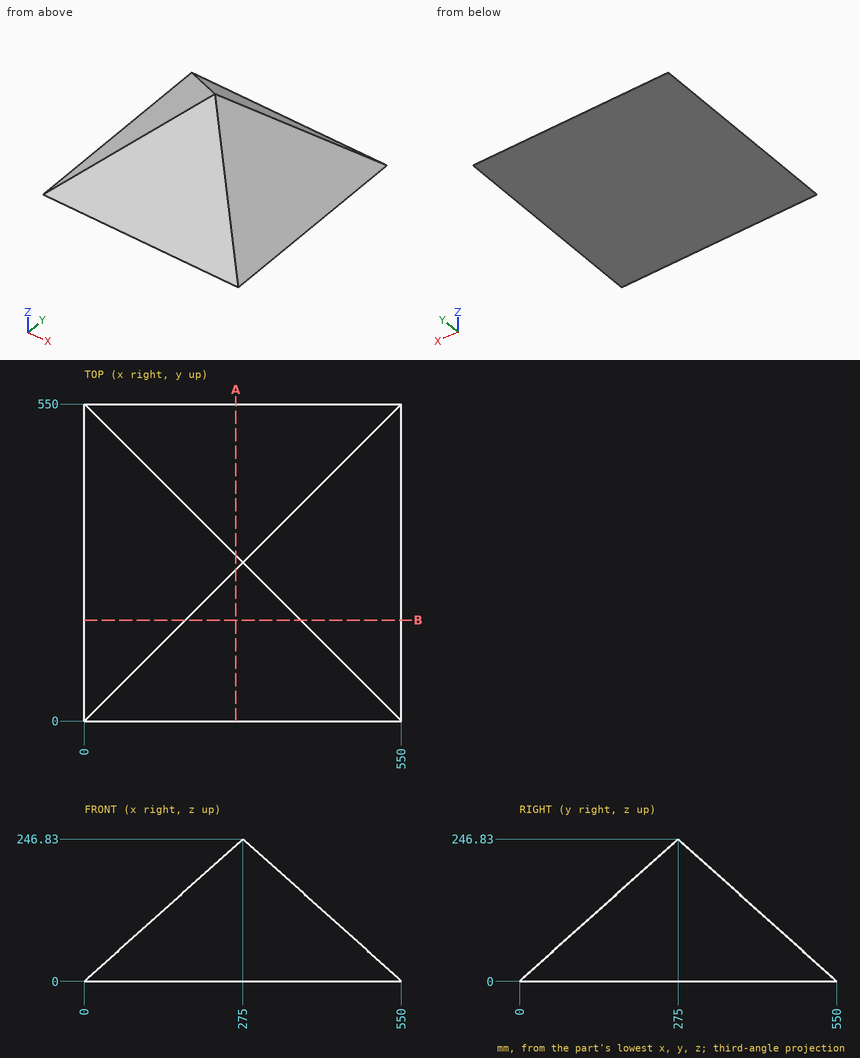
Could you check a few things on this drawing? It's one solid part, dimensions in mm from its lowest x, y, z. Give positions to 0.01 mm unless a question says otherwise; leave off trailing zeros. Write each loop counter-clockwise with the first axis right and the second up, starting at its lowest first coordinate (ties: lowest second). Pieces come first, ordered by that corner, then holes. Notation, with made-up numbers: (69, 57.5) -> (107, 57.5) arc R22 ccw to (107, 64.5) -> close; hole circle Ø8 at (-31.75, 85). An arc over 180 degrees is marked (long way). Write item = value, one per line.
(1) Suppose I cut it at A-A on x = 262.5. Write out the boundary of the cut face in (y, z), then the cut area to 3 significant figures.
Worked out:
outline = (0, 0) -> (550, 0) -> (287.5, 235.61) -> (262.5, 235.61) -> close
area = 67,700 mm^2
(2) I'm going to push flat-ended pins straight in: P1, Ø3, axis at x = 270, y = 366, coming from the +Z side; P2, Ø2, axis at y = 277.5, z = 218, coming from the -X side; P3, Ø6, axis at y = 286, z = 154, coming from the +X side. Where does each tip first touch, or does it pass through?
Worked out:
P1 = 166.5
P2 = 241.77
P3 = 381.77
(3) Suppose I cut it at B-B on y = 175. Write out the boundary of the cut face in (x, z).
Worked out:
outline = (0, 0) -> (550, 0) -> (375, 157.07) -> (175, 157.07) -> close
(4) I need wall thicknesses on probe 1 along Y at (x, z) = (177.5, 127); probe 2 along Z at (x, y) = (503.5, 255.5); probe 3 along Y at (x, z) = (290.5, 194). Which ranges of each line are inside material? Lowest first, please. Write a range as from..to.
Worked out:
probe_1 = 141.49..408.51
probe_2 = 0..41.74
probe_3 = 216.14..333.86
